For this review, take the finished solid that the model builds, in its own axes (mm). Face numbers are marked on the shaded views. Coordinates: 2 decimals unless noted, no trailing zeros. Write item = value, one per line. Start each with the question number.
1) Wall thickness on probe 1 along X at (y, z) = (-0.2, -0.25); probe 2 along Y at (x, z) = (-8.5, -0.75); probe 3 along X at (y, z) = (-0.2, -2.5): over which ranges is each line inside the solid? List them lowest first. Write a range as [from, to].
2) Insertion check: pin 1 Ø10 at (x, z) = (-2, 5.5) entering from -Y; pin 2 Ø1 at (y, z) = (2, 6) entering from +X; pin 3 Ø0.9 at (x, y) = (0, -1.5) entering from +Z; pin 4 Ø0.5 at (x, y) = (0, -1) entering from -Z. Each pin has a flat end and moves straight along its axis. Give the tip position at first contact, or say it passes through.
3) Consider section B-B on x = 0. State how many separate pieces and enclosed holes the cut face has, and give its area (3 significant figures).
4) Draft analysis for pull direction X (two halves, no side actions). For the marked faces 1 and 2, state which applies: +X half, -X half, draft (parallel to the pull), parting line (faces both ways), or undercut.
from build123d import *

# Parameters (mm, degrees)
F4_W          = 1.0840747273
F4_H          = 19.680833444
F5_DEPTH      = 25
F5_DEPTH_BACK = 25


# Not quite as in the source:
# - a fillet or chamfer that OpenCascade refuses, or shapes differently, is made with other operations: its cross-section is extruded or revolved along the edge and cut away or added


with BuildPart() as f2:
    # F2: sweep along a path in F0
    with BuildLine(Plane.XZ) as f2_path:
        CenterArc((0, 0), 8.65, 0, 360)
    # F1 (on Right) → F2 (sweep)
    with BuildSketch(Plane.YZ):
        Polygon((-2.5, 8.4675319269), (0, 8.4675319269), (2.5, 8.4675319269), (2.6424242295, 10.246030055), (0.5, 10.7327634469), (0.5, 9.5877971399), (0.344154765, 9.4675319269), (0, 9.4675319269), (-0.344154765, 9.4675319269), (-0.5, 9.5877971399), (-0.5, 10.7327634469), (-2.6424242295, 10.246030055), align=None)
    sweep(path=f2_path.line)

    # F3: fillet of radius 2.0708896165 on 2 edges, made by hand

    # F3_s1 → F3_t2 (revolve, cut)
    with BuildSketch(Plane.XY):
        with BuildLine():
            ThreePointArc((8.4585593646, -2.4992814666), (9.85018085, -2.103755641), (10.6432988419, -0.8937908116))
            Line((10.6432988419, -0.8937908116), (10.246030055, -2.6424242295))
            Line((10.246030055, -2.6424242295), (8.4585593646, -2.4992814666))
        make_face()
    revolve(axis=Axis((0, -2.6424242295, 0), (0, -1, 0)), mode=Mode.SUBTRACT)

    # F3_s3 → F3_t4 (revolve, cut)
    with BuildSketch(Plane.XY):
        with BuildLine():
            ThreePointArc((8.4585593646, 2.4992814666), (9.85018085, 2.103755641), (10.6432988419, 0.8937908116))
            Line((10.6432988419, 0.8937908116), (10.246030055, 2.6424242295))
            Line((10.246030055, 2.6424242295), (8.4585593646, 2.4992814666))
        make_face()
    revolve(axis=Axis((0, 2.6424242295, 0), (0, -1, 0)), mode=Mode.SUBTRACT)

    # F4 (on Front) → F5 (cut, two sides)
    with BuildSketch(Plane.XZ) as f5_sk:
        Rectangle(F4_W, F4_H)
    extrude(amount=-F5_DEPTH, mode=Mode.SUBTRACT)
    extrude(f5_sk.sketch, amount=F5_DEPTH_BACK, mode=Mode.SUBTRACT)


solid = f2.part
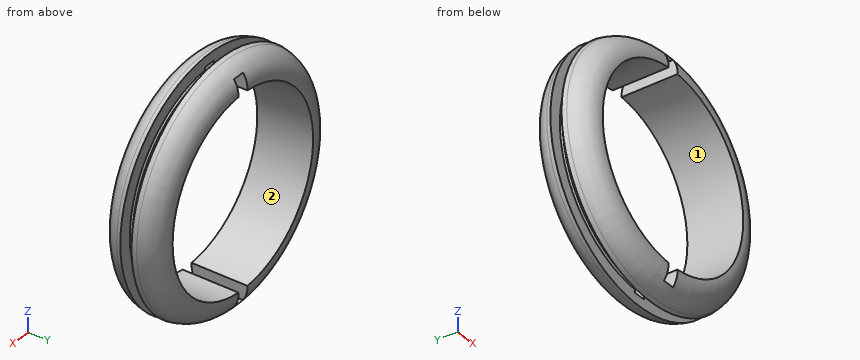
Answer sheet:
q1.probe_1 = [-9.46, -8.46], [8.46, 9.46]
q1.probe_2 = [-2.5, 2.5]
q1.probe_3 = [-9.13, -8.09], [8.09, 9.13]
q2.pin_1 = -2.51
q2.pin_2 = 8.62
q2.pin_3 = 10.6
q2.pin_4 = -10.68
q3.separate_pieces = 4
q3.enclosed_holes = 0
q3.area = 3.81 mm2
q4.face_1 = undercut
q4.face_2 = undercut
